Verification items for the finished model (mm, model axes). A direction names the side the tool comes from. Give positions to 0.01 mm unless a question says otherwise; leave off trailing zeros. Loops run counter-clockwise (first coordinate to the right, second up) from the corner with the lowest first, then second, coordinate; pieces in that order, holes last. Notation, with made-up numbers: M -1.5,-16 L 40.5,-16 A13 cw 40.5,8 Z; hole C 78,-39 d5. An arc over 180 degrees is marked long. Answer in a Markdown table with one row per item.
```python
from build123d import *

# Parameters (mm, degrees)
BOSS_EXTRUDE1_DEPTH = 31.75


with BuildPart() as part:
    # Sketch2 → Boss-Extrude1 (new, symmetric)
    with BuildSketch(Plane.XY):
        with BuildLine():
            Line((-25.4, 50.8), (-38.1, 50.8))
            Line((-38.1, 50.8), (-38.1, 12.7))
            Line((-38.1, 12.7), (-76.2, 12.7))
            Line((-76.2, 12.7), (-76.2, 0))
            Line((-76.2, 0), (76.2, 0))
            Line((76.2, 0), (76.2, 12.7))
            Line((76.2, 12.7), (38.1, 12.7))
            Line((38.1, 12.7), (38.1, 50.8))
            Line((38.1, 50.8), (25.4, 50.8))
            ThreePointArc((25.4, 50.8), (0, 25.4), (-25.4, 50.8))
        make_face()
    extrude(amount=BOSS_EXTRUDE1_DEPTH, both=True)


solid = part.part
```
Item 1: Sectioned sample at C-C (x = -49.5). Record the cut outline in (y, z), and give its area (3 significant figures).
Reported:
| item | result |
|---|---|
| outline | M 0,-31.75 L 12.7,-31.75 L 12.7,31.75 L 0,31.75 Z |
| area | 806 mm^2 |
Item 2: Sectioned sample at D-D (y = 18.5). Record the cut outline in (x, z).
Reported:
| item | result |
|---|---|
| outline | M -38.1,-31.75 L 38.1,-31.75 L 38.1,31.75 L -38.1,31.75 Z |
Item 3: Scan lines: L1, parallel to X at y = 38, z = 7.5; L2, parallel to X at y = 36, z = -28; L3, parallel to Y at x = 1, z = 22. Record each from-to range of solid material in increasing order. Write a range as [from, to].
Reported:
| item | result |
|---|---|
| L1 | x = [-38.1, -21.94], [21.94, 38.1] |
| L2 | x = [-38.1, -20.64], [20.64, 38.1] |
| L3 | y = [0, 25.42] |
Item 4: Go/stop test with flat-tipped pins: pin 1 (19 mm diameter, centred on y = 36, z = -13, fed in from -X); pin 2 (6 mm diameter, centred on y = 39.5, z = 23, fed in from +X); pin 3 (19 mm diameter, centred on x = 58, z = 8, fed in from +Y). Record where each tip stops, or that it passes through.
Reported:
| item | result |
|---|---|
| pin 1 | stops at x = -38.1 |
| pin 2 | stops at x = 38.1 |
| pin 3 | stops at y = 12.7 |
Item 5: Sectioned sample at B-B (y = 40.5). Record the cut outline in (x, z).
Reported:
| item | result |
|---|---|
| outline | M -38.1,-31.75 L -23.22,-31.75 L -23.22,31.75 L -38.1,31.75 Z; M 23.22,-31.75 L 38.1,-31.75 L 38.1,31.75 L 23.22,31.75 Z |
Item 6: Release check for a two-part mould opening along X. For faces 1 (the flat face through (-1, 0, 0)), 2 (the flat face through (-38.1, 32, 0)), 3 (the cylindrical face through (0.559, 25.406, 0.444)) record: released by +X, released by -X, zero draft, split by the parting line, or undercut.
Reported:
| item | result |
|---|---|
| face 1 | zero draft |
| face 2 | released by -X |
| face 3 | undercut |
Item 7: Tool access check on faces 4 (the flat face through (38.1, 31, 0)), 5 (the flat face through (-57, 12.7, 0)), 6 (the flat face through (-76.2, 6, 0)). Record the directions out of +Z, -Z, +X, -X, +Y, -Y that give a thin tool (end or side, any length) a straight path to the whole face; none if there is none.
Reported:
| item | result |
|---|---|
| face 4 | +Z, -Z, +X, +Y |
| face 5 | +Z, -Z, -X, +Y |
| face 6 | +Z, -Z, -X, +Y, -Y |
Item 8: Sectioned sample at A-A (z = 1). Record the cut outline in (x, y), and give its area (3 significant figures).
Reported:
| item | result |
|---|---|
| outline | M -76.2,0 L 76.2,0 L 76.2,12.7 L 38.1,12.7 L 38.1,50.8 L 25.4,50.8 A25.4 cw -25.4,50.8 L -38.1,50.8 L -38.1,12.7 L -76.2,12.7 Z |
| area | 3,830 mm^2 |
